Source: CAD feature listing. Evaluate the final solid. Frame: model axes, mm. Face numbers are marked on the shaded views. Coordinates: 2 decimals unless noted, no trailing zeros. Order: outer loops, then holes, each group sorted by start corner. A loop starts at its lowest first (then second) coordinate and runs counter-clockwise, first axis right, second up.
Item 1: Section D-D on x = 5.5. Return the cut outline in (y, z) (3 decimals), then the cut area to 3 significant figures.
Item 2: Section A-A on z = 0. State how many separate pieces and enclosed holes the cut face has, then the cut area to 3 significant figures.
Item 3: Ray query, line 1 (X direction, y = 2.35, z = 0); line 2 (X direction, y = 1.6, z = 0); line 3 (Z direction, x = -8.5, y = 1.4). Return the intervals inside material, ascending.
Item 4: Section B-B on x = 0. Return the cut outline in (y, z) (3 decimals).
Item 5: Contact query for flat-ended pins moving along their axis: P1, Ø3, axis at x = -7.44, z = 0, coming from the +Y side; P2, Ø4, axis at x = -2.5, z = -2, coming from the -Y side; P3, Ø3.5, axis at x = 22.225, z = 0, coming from the +Y side. Output: stop coordinate, or through.
Item 6: Mould query, pull axis Z, two halves, no side actions, for the marked faces 1, 2, 3 and 4. Classes: released by +Z, released by -Z, zero draft, split by the parting line, or undercut.
Item 7: Section C-C on y = 1.05. Return the cut outline in (x, z) (3 decimals).
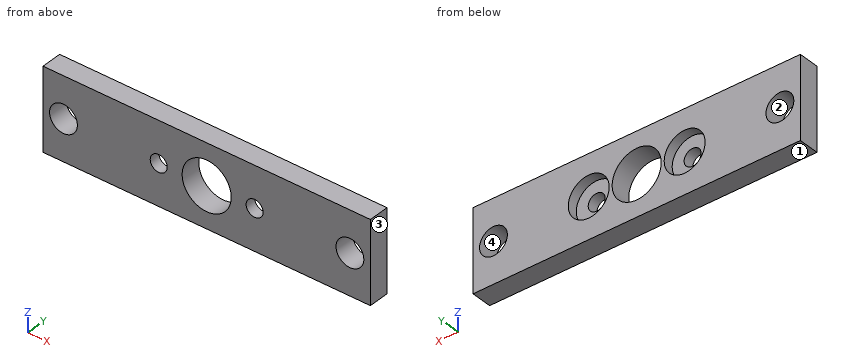
from build123d import *

# Parameters (mm, degrees)
SKETCH1_W           = 50.8
SKETCH1_H           = 12.7
SKETCH1_R           = 3.81
SKETCH1_R_2         = 1.3208
SKETCH1_R_3         = 2.159
BOSS_EXTRUDE1_DEPTH = 3.175
SKETCH2_R           = 3.175
CUT_EXTRUDE1_DEPTH  = 1.524


with BuildPart() as part:
    # Sketch1 → Boss-Extrude1 (new body)
    with BuildSketch(Plane(origin=(0, 0, 0), x_dir=(1, 0, 0), z_dir=(0, 1, 0))):
        Rectangle(SKETCH1_W, SKETCH1_H)
        with Locations(Location((0, 0, 0), (0, 0, 270))):
            Circle(SKETCH1_R, mode=Mode.SUBTRACT)
        with Locations(Location((7.4422, 0, 0), (0, 0, 270))):
            Circle(SKETCH1_R_2, mode=Mode.SUBTRACT)
        with Locations(Location((-7.4422, 0, 0), (0, 0, 270))):
            Circle(SKETCH1_R_2, mode=Mode.SUBTRACT)
        with Locations(Location((-22.225, 0, 0), (0, 0, 270))):
            Circle(SKETCH1_R_3, mode=Mode.SUBTRACT)
        with Locations(Location((22.225, 0, 0), (0, 0, 270))):
            Circle(SKETCH1_R_3, mode=Mode.SUBTRACT)
    extrude(amount=BOSS_EXTRUDE1_DEPTH)

    # Sketch2 → Cut-Extrude1 (cut)
    with BuildSketch(Plane(origin=(0, 3.175, 0), x_dir=(1, 0, 0), z_dir=(0, 1, 0))):
        with Locations(Location((-7.4422, 0, 0), (0, 0, 270))):
            Circle(SKETCH2_R)
        with Locations(Location((7.4422, 0, 0), (0, 0, 270))):
            Circle(SKETCH2_R)
    extrude(amount=-CUT_EXTRUDE1_DEPTH, mode=Mode.SUBTRACT)


solid = part.part
Answer list:
1. outline: (0, -6.35) - (3.175, -6.35) - (3.175, -2.512) - (1.651, -2.512) - (1.651, 2.512) - (3.175, 2.512) - (3.175, 6.35) - (0, 6.35) - close
1. area: 32.7 mm2
2. separate pieces: 6
2. enclosed holes: 0
2. area: 81.6 mm2
3. line 1: x = -25.4 to -24.38, -20.07 to -10.62, -4.27 to -3.81, 3.81 to 4.27, 10.62 to 20.07, 24.38 to 25.4
3. line 2: x = -25.4 to -24.38, -20.07 to -8.76, -6.12 to -3.81, 3.81 to 6.12, 8.76 to 20.07, 24.38 to 25.4
3. line 3: z = -6.35 to -0.79, 0.79 to 6.35
4. outline: (0, -6.35) - (3.175, -6.35) - (3.175, -3.81) - (0, -3.81) - close; (0, 3.81) - (3.175, 3.81) - (3.175, 6.35) - (0, 6.35) - close
5. P1: stops at y = 1.65
5. P2: stops at y = 0
5. P3: passes through
6. face 1: released by -Z
6. face 2: undercut
6. face 3: zero draft
6. face 4: undercut
7. outline: (-25.4, -6.35) - (25.4, -6.35) - (25.4, 6.35) - (-25.4, 6.35) - close; hole circle Ø4.318 at (-22.225, 0); hole circle Ø2.642 at (-7.442, 0); hole circle Ø7.62 at (0, 0); hole circle Ø2.642 at (7.442, 0); hole circle Ø4.318 at (22.225, 0)
